The model under review builds one solid part; all positions refer to its coordinate system, in mm. Coordinates: 2 decimals unless noted, no trailing zeros. Order: outer loops, then holes, each group sorted by start corner. A loop starts at its lowest first (then second) coordinate and runs counter-clockwise, first axis right, second up. Notation, with made-up numbers: (14, -12) -> (63, -12) arc R16 ccw to (63, -4) -> close; hole circle Ø4 at (82, 55). An arc over 180 degrees is marked (long way). Use one line per item in the form item = value. Start each with the question number.
(1) Take a section at B-B (y = 13). State the section outline as (x, z) points, then the cut area to 3 significant figures.
(2) Take a section at A-A (x = -19.75). State the section outline as (y, z) points, then the cut area to 3 significant figures.
(3) Mouldability with a two-part tool opening along X and no side actions: class faces 1 (the cylindrical face through (14.76, -14.91, 1.48)), 2 (the cylindrical face through (22.65, 19.43, 1.52)), 3 (the cylindrical face through (-18.57, -11.92, 1.48)), 4 (the flat face through (0, 0, 3)) as +X half, -X half, draft (parallel to the pull), parting line (faces both ways), or undercut.
(4) Wall thickness on line 1 along Y through (x, z) = (15.75, 1.7); line 2 along Y through (x, z) = (-19.75, 0.75); line 3 along X through (y, z) = (12, 2.5): over which ranges is each line inside the solid? List them lowest first.
(5) Take a section at C-C (z = 2.55). State the section outline as (x, y) points, then the cut area to 3 significant figures.
```python
from build123d import *

# Parameters (mm, degrees)
SKETCH1_W                = 46.5
SKETCH1_H                = 40
BOSS_EXTRUDE1_DEPTH      = 3
M3_CLEARANCE_HOLE1_D     = 3.2
M3_CLEARANCE_HOLE1_DEPTH = 8
M3_CLEARANCE_HOLE1_TIP   = 0.96137699
M4_CLEARANCE_HOLE1_D     = 4.3
M4_CLEARANCE_HOLE1_DEPTH = 8
M4_CLEARANCE_HOLE1_TIP   = 1.291850331
FILLET1_R                = 2


with BuildPart() as part:
    # Sketch1 → Boss-Extrude1 (new body)
    with BuildSketch(Plane.XY):
        Rectangle(SKETCH1_W, SKETCH1_H)
    extrude(amount=BOSS_EXTRUDE1_DEPTH)

    # M3 Clearance Hole1
    with Locations(Plane.XY.offset(3)):
        with Locations((-19.75, 13), (-19.75, -13)):
            Hole(M3_CLEARANCE_HOLE1_D / 2, depth=M3_CLEARANCE_HOLE1_DEPTH)
            with Locations((0, 0, -(M3_CLEARANCE_HOLE1_DEPTH + M3_CLEARANCE_HOLE1_TIP / 2))):  # 118° drill point
                Cone(0, M3_CLEARANCE_HOLE1_D / 2, M3_CLEARANCE_HOLE1_TIP, mode=Mode.SUBTRACT)

    # M4 Clearance Hole1
    with Locations(Plane.XY.offset(3)):
        with Locations((15.75, 13), (15.75, -13)):
            Hole(M4_CLEARANCE_HOLE1_D / 2, depth=M4_CLEARANCE_HOLE1_DEPTH)
            with Locations((0, 0, -(M4_CLEARANCE_HOLE1_DEPTH + M4_CLEARANCE_HOLE1_TIP / 2))):  # 118° drill point
                Cone(0, M4_CLEARANCE_HOLE1_D / 2, M4_CLEARANCE_HOLE1_TIP, mode=Mode.SUBTRACT)

    # Fillet1
    fillet1_edges = [part.edges().sort_by_distance(p)[0] for p in [
        (-23.25, 20, 1.5),
        (23.25, 20, 1.5),
        (23.25, -20, 1.5),
        (-23.25, -20, 1.5),
    ]]
    fillet(fillet1_edges, radius=FILLET1_R)


solid = part.part
```
Findings:
q1.outline = (-23.25, 0) -> (-21.35, 0) -> (-21.35, 3) -> (-23.25, 3) -> close; (-18.15, 0) -> (13.6, 0) -> (13.6, 3) -> (-18.15, 3) -> close; (17.9, 0) -> (23.25, 0) -> (23.25, 3) -> (17.9, 3) -> close
q1.area = 117 mm²
q2.outline = (-20, 0) -> (-14.6, 0) -> (-14.6, 3) -> (-20, 3) -> close; (-11.4, 0) -> (11.4, 0) -> (11.4, 3) -> (-11.4, 3) -> close; (14.6, 0) -> (20, 0) -> (20, 3) -> (14.6, 3) -> close
q2.area = 101 mm²
q3.face_1 = undercut
q3.face_2 = +X half
q3.face_3 = undercut
q3.face_4 = draft
q4.line_1 = -20 to -15.15, -10.85 to 10.85, 15.15 to 20
q4.line_2 = -20 to -14.6, -11.4 to 11.4, 14.6 to 20
q4.line_3 = -23.25 to -21, -18.5 to 13.85, 17.65 to 23.25
q5.outline = (-23.25, -18) arc R2 ccw to (-21.25, -20) -> (21.25, -20) arc R2 ccw to (23.25, -18) -> (23.25, 18) arc R2 ccw to (21.25, 20) -> (-21.25, 20) arc R2 ccw to (-23.25, 18) -> close; hole circle Ø3.2 at (-19.75, -13); hole circle Ø3.2 at (-19.75, 13); hole circle Ø4.3 at (15.75, -13); hole circle Ø4.3 at (15.75, 13)
q5.area = 1,810 mm²
